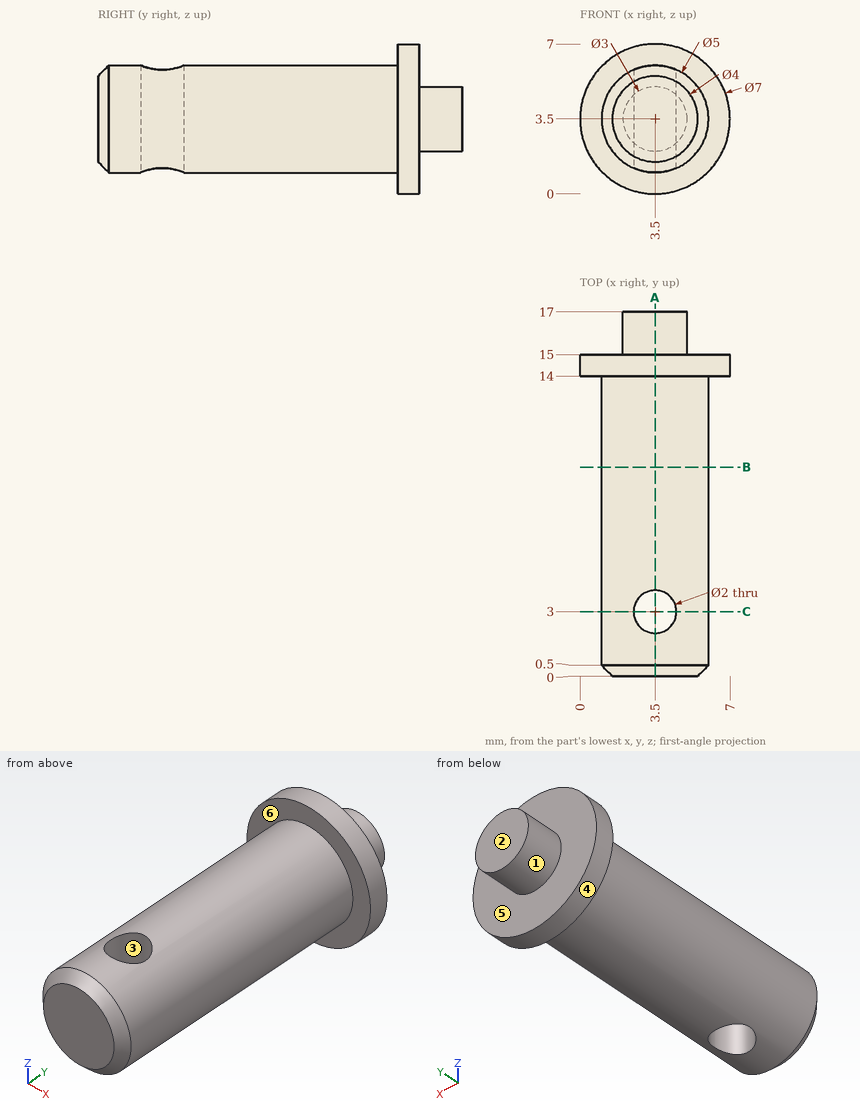
For this review, use the dimensioned drawing (mm, ordinates from the lowest corner) and the shaded views. A direction names the side the tool comes from. Round coordinates to 2 decimals unless told otherwise and drop trailing zeros. Write each loop counter-clockwise with the first axis right and the second up, starting at its lowest first coordinate (ties: lowest second). Pieces come first, ordered by that corner, then holes. Notation, with made-up numbers: (-6.75, 80) -> (19.25, 80) arc R33 ccw to (19.25, 108) -> close; hole circle Ø4 at (-37, 23). An arc over 180 degrees is marked (long way). Use CSV: the item, a comma, the result in double quotes.
(1) Clearance check with flat-ended pins moving along their axes: P1, Ø3, axis at x = 1, y = 9.5, coming from the -Z side; P2, Ø2, axis at x = 5, y = 11.5, coming from the -Z side; P3, Ø2.5, axis at x = 3.5, y = 3, coming from the -Z side. State where each tip first meets the part, or that it passes through.
Computed values:
P1,"z = 1.21"
P2,"z = 1.05"
P3,"z = 1"
(2) Consider section B-B, the plane y = 9.75. Give the boundary of the cut face in (x, z), plus the area to 3 significant figures.
Computed values:
outline,"circle Ø5 at (3.5, 3.5)"
area,"19.6 mm²"
(3) Consider section A-A, the plane x = 3.5. Give the boundary of the cut face in (y, z), plus the area to 4 significant figures.
Computed values:
outline,"(0, 1.5) -> (0.5, 1) -> (2, 1) -> (2, 6) -> (0.5, 6) -> (0, 5.5) -> close; (4, 1) -> (14, 1) -> (14, 0) -> (15, 0) -> (15, 2) -> (17, 2) -> (17, 5) -> (15, 5) -> (15, 7) -> (14, 7) -> (14, 6) -> (4, 6) -> close"
area,"72.75 mm²"
(4) Consider section C-C, the plane y = 3. Give the boundary of the cut face in (x, z), plus the area to 3 significant figures.
Computed values:
outline,"(2.5, 1.21) -> (2.5, 5.79) arc R2.5 ccw to start; (4.5, 1.21) arc R2.5 ccw to (4.5, 5.79) -> close"
area,"9.91 mm²"
(5) For the marked faces 4, 5 and 6, list the 3-axis set-ups (+Z, -Z, +X, -X, +Y, -Y) from which the entire face can be reached by the end or side of a thin tool; tool diameter is ignored.
Computed values:
face 4,"+Y, -Y"
face 5,"+Y"
face 6,"-Y"
(6) Draft analysis for pull direction X (two halves, no side actions). For the marked faces 1, 2 and 3, state which applies: +X half, -X half, draft (parallel to the pull), parting line (faces both ways), or undercut.
Computed values:
face 1,"parting line"
face 2,"draft"
face 3,"undercut"
(7) To check wall thickness, follow L1, parallel to Y at x = 3.5, z = 3.2; L2, parallel to Y at x = 3.5, z = 0.75; L3, parallel to X at y = 4.75, z = 1.5. State the ranges of each line that lie inside material, in increasing order. Write a range as [from, to].
Computed values:
L1,"[0, 2], [4, 17]"
L2,"[14, 15]"
L3,"[2, 5]"
